```python
from build123d import *

# Parameters (mm, degrees)
SKETCH1_W           = 15
SKETCH1_H           = 12
SKETCH1_W_2         = 10
SKETCH1_H_2         = 8
BOSS_EXTRUDE1_DEPTH = 1.5
BOSS_EXTRUDE2_REACH = 12
SKETCH2_R           = 1.5
CHAMFER1_SIZE       = 2
CHAMFER2_SIZE       = 2


with BuildPart() as part:
    # Sketch1 → Boss-Extrude1 (new body, symmetric)
    with BuildSketch(Plane(origin=(0, 0, 0), x_dir=(1, 0, 0), z_dir=(0, 1, 0))):
        Rectangle(SKETCH1_W, SKETCH1_H)
        Rectangle(SKETCH1_W_2, SKETCH1_H_2, mode=Mode.SUBTRACT)
    extrude(amount=BOSS_EXTRUDE1_DEPTH, both=True)

    # Sketch2 → Boss-Extrude2 (add, up to next)
    with BuildSketch(Plane.XY.offset(-4), mode=Mode.PRIVATE) as boss_extrude2_sk1:
        Circle(SKETCH2_R)
    boss_extrude2_tool1 = extrude(boss_extrude2_sk1.sketch, amount=BOSS_EXTRUDE2_REACH, mode=Mode.PRIVATE) - part.part
    add(boss_extrude2_tool1.solids().sort_by_distance((0, 0, -4))[0])

    # Chamfer1
    chamfer1_edges = [part.edges().sort_by_distance(p)[0] for p in [
        (5, -1.5, 0),
    ]]
    chamfer(chamfer1_edges, length=CHAMFER1_SIZE)

    # Chamfer2
    chamfer2_edges = [part.edges().sort_by_distance(p)[0] for p in [
        (-5, 1.5, 0),
    ]]
    chamfer(chamfer2_edges, length=CHAMFER2_SIZE)


solid = part.part
```
Work out the finished part from the listing and answer in its coordinate system (mm). A direction names the side the tool comes from. Give positions to 0.01 mm unless a question says otherwise; leave off trailing zeros. Order: outer loops, then holes, each group sorted by start corner. A loop starts at its lowest first (then second) coordinate and runs counter-clockwise, first axis right, second up. Notation, with made-up numbers: (32.25, 61) - (50.25, 61) arc R17 ccw to (50.25, 80) - close; hole circle Ø1 at (-8, 67). An arc over 180 degrees is marked (long way). One line per item, written item: value. Start each with the question number.
1. Section C-C, the plane y = 0 is taken. Write down the section's boundary in (x, z), then the cut area to 3 significant figures.
2. This flat-tipped pin is pushed along its axis until it touches: pin 1 Ø1 at (x, z) = (3, 1.5) entering from +Y. Where does it stop, or does it pass through?
3. Which of the six approach directions +Z, -Z, +X, -X, +Y, -Y give full straight-line access (tool end or side, diameter ignored) to faces 5 (the face through (-1.5, 0.07, -0.06)), 6 (the face through (2, 1.5, -5)), 7 (the face through (5, 1, 0))?
4. For a pull along X with two mould halves and no side action, classify faces 1 (the face through (7.5, 0, 0)), 2 (the face through (0, 0, 6)), 3 (the face through (-6, 0.5, 0.1)), 4 (the face through (6, -0.5, 0.1)) as released by +X, released by -X, zero draft, split by the parting line, or undercut.
5. Consider line 1 (Z direction, x = 3.5, y = 1.4); line 2 (X direction, y = 0, z = 3.5); line 3 (X direction, y = -1, z = -2.25). Determine where each line is inside the solid, lowest interval first.
6. Section D-D, the plane x = 5.5 is taken. Write down the section's boundary in (y, z), then the cut area to 3 significant figures.
7. Section B-B, the plane z = -1.5 is taken. Write down the section's boundary in (x, y).
8. Section A-A, the plane x = -4 is taken. Write down the section's boundary in (y, z).
Filled sheet:
1. outline: (-7.5, -6) - (7.5, -6) - (7.5, 6) - (-7.5, 6) - close; hole (-5.5, -4) - (-1.5, -4) - (-1.5, 4) - (-5.5, 4) - close; hole (1.5, -4) - (5.5, -4) - (5.5, 4) - (1.5, 4) - close
1. area: 116 mm²
2. pin 1: through
3. face 5: none
3. face 6: +Z, -Z, +X, -X, +Y
3. face 7: +Y, -Y
4. face 1: released by +X
4. face 2: zero draft
4. face 3: undercut
4. face 4: undercut
5. line 1: -6 to -4, 4 to 6
5. line 2: -7.5 to -5.5, -1.5 to 1.5, 5.5 to 7.5
5. line 3: -7.5 to -5, -1.12 to 1.12, 6.5 to 7.5
6. outline: (-1.5, -6) - (1.5, -6) - (1.5, 6) - (-1.5, 6) - (-1.5, 4) - (0, 4) - (0, -4) - (-1.5, -4) - close
6. area: 24.0 mm²
7. outline: (-7.5, -1.5) - (-5, -1.5) - (-5, -0.5) - (-7, 1.5) - (-7.5, 1.5) - close; circle Ø3 at (0, 0); (5, 0.5) - (7, -1.5) - (7.5, -1.5) - (7.5, 1.5) - (5, 1.5) - close
8. outline: (-1.5, -6) - (1.5, -6) - (1.5, -4) - (-1.5, -4) - close; (-1.5, 4) - (1.5, 4) - (1.5, 6) - (-1.5, 6) - close
